from build123d import *

# Parameters (mm, degrees)
F1_DEPTH      = 9
F3_DEPTH      = 25
F4_R          = 4.5
F4_R_2        = 3.5
F5_DEPTH      = 24
F7_DEPTH      = 25
F7_DEPTH_BACK = 25


with BuildPart() as f1:
    # F0 (on Top) → F1 (new body)
    with BuildSketch(Plane.XY):
        Polygon((-3.3, 3.3), (-3.3, 0), (-3.3, -3.3), (0, -3.3), (3.3, -3.3), (3.3, 0), (3.3, 3.3), (0, 3.3), align=None)
        Polygon((6.6, -3.810512), (6.6, 3.810512), (0, 7.621024), (-6.6, 3.810512), (-6.6, -3.810512), (0, -7.621024), align=None)
        Polygon((-3.3, -3.3), (-3.3, 0), (-3.3, 3.3), (0, 3.3), (3.3, 3.3), (3.3, 0), (3.3, -3.3), (0, -3.3), align=None, mode=Mode.SUBTRACT)
    extrude(amount=F1_DEPTH)

    # F2 (on face) → F3 (cut)
    with BuildSketch(Plane(origin=(-6.6, 0, 0), x_dir=(0, -1, 0), z_dir=(-1, 0, 0))):
        with BuildLine():
            ThreePointArc((1.6, -12), (1.131371, -10.868629), (0, -10.4))
            ThreePointArc((0, -10.4), (-1.131371, -13.131371), (1.6, -12))
        make_face()
    extrude(amount=-F3_DEPTH, mode=Mode.SUBTRACT)

    # F4 (on face) → F5 (join)
    with BuildSketch(Plane(origin=(0, 0, 0), x_dir=(1, 0, 0), z_dir=(0, 0, -1))):
        Circle(F4_R)
        Circle(F4_R_2, mode=Mode.SUBTRACT)
    extrude(amount=F5_DEPTH)

    # F6 (on face) → F7 (cut, two sides)
    with BuildSketch(Plane(origin=(0, -3.3, 0), x_dir=(-1, 0, 0), z_dir=(0, 1, 0))) as f7_sk:
        with BuildLine():
            ThreePointArc((0, -16.4), (-1.131371, -19.131371), (1.6, -18))
            ThreePointArc((1.6, -18), (1.131371, -16.868629), (0, -16.4))
        make_face()
    extrude(amount=F7_DEPTH, mode=Mode.SUBTRACT)
    extrude(f7_sk.sketch, amount=-F7_DEPTH_BACK, mode=Mode.SUBTRACT)


solid = f1.part
Model file for the job. Use its own axes, mm. A direction names the side the tool comes from. Coordinates: 2 decimals unless noted, no trailing zeros. Loops run counter-clockwise (first coordinate to the right, second up) from the corner with the lowest first, then second, coordinate; pieces in that order, holes last. Notation, with made-up numbers: (84.25, -17.75) -> (98.25, -17.75) arc R8 cw to (98.25, -12.75) -> close; hole circle Ø11 at (-20.5, 19.25). An arc over 180 degrees is marked (long way). Use one line per item in the form item = value. Start each with the question number.
(1) Cut at C-C on x = -0.5. Give the cut face in (y, z), and give its area (3 significant figures).
(2) Cut at D-D on y = 2.75. Give the cut face in (x, z), and give its area (3 significant figures).
(3) Cut at B-B on z = 4.5. Give the cut face in (x, y).
(4) Flat gauge pins, fed straight in: pin 1 (4 mm diameter, centred on x = 0, y = -2, fed in from -Z); pin 2 (4 mm diameter, centred on x = -3.5, z = -8.5, fed in from -Y); pin 3 (5 mm diameter, centred on x = 0, z = -18, fed in from -Y); pin 4 (8 mm diameter, centred on y = 4, z = -9.5, fed in from +X). Where does each tip first touch, or does it go through?
(5) Tool access for faces 5 (the flat face through (3.3, 0, 4)), 6 (the cylindrical face through (4.292, -1.352, -11.832)), 7 (the flat face through (3.254, -5.742, 4.437)): list every direction of +Z, -Z, +X, -X, +Y, -Y with a clear straight run to the whole face (end or side of a thin tool).
(6) Probe probe 1 along X at (y, z) = (0, -4); probe 2 along X at (y, z) = (1, 3). List the from-to ranges inside material, lowest first. Write a range as from..to.
(7) Cut at A-A on y = 0. Give the cut face in (x, z).
(8) Pull direction X, two halves, no side cores. Call faces 1 (the flat face through (-3.254, 5.742, 4.437)), 2 (the flat face through (3, 3, 0)), 3 (the flat face through (6.6, 0, 4)), 4 (the flat face through (0, 4, -24)): pulls with the +X half, pulls with the -X half, needs draft (parallel to the pull), parting line crosses it, or undercut.
Values:
q1.outline = (-7.33, 0) -> (-4.47, 0) -> (-4.47, -16.48) -> (-3.46, -16.48) -> (-3.46, 0) -> (-3.3, 0) -> (-3.3, 9) -> (-7.33, 9) -> close; (-4.47, -24) -> (-3.46, -24) -> (-3.46, -19.52) -> (-4.47, -19.52) -> close; (3.3, 0) -> (3.46, 0) -> (3.46, -16.48) -> (4.47, -16.48) -> (4.47, 0) -> (7.33, 0) -> (7.33, 9) -> (3.3, 9) -> close; (3.46, -24) -> (4.47, -24) -> (4.47, -19.52) -> (3.46, -19.52) -> close
q1.area = 115 mm2
q2.outline = (-6.6, 0) -> (-3.56, 0) -> (-3.56, -24) -> (-2.17, -24) -> (-2.17, 0) -> (-3.3, 0) -> (-3.3, 9) -> (-6.6, 9) -> close; (2.17, -24) -> (3.56, -24) -> (3.56, 0) -> (6.6, 0) -> (6.6, 9) -> (3.3, 9) -> (3.3, 0) -> (2.17, 0) -> close
q2.area = 126 mm2
q3.outline = (-6.6, -3.81) -> (0, -7.62) -> (6.6, -3.81) -> (6.6, 3.81) -> (0, 7.62) -> (-6.6, 3.81) -> close; hole (-3.3, -3.3) -> (3.3, -3.3) -> (3.3, 3.3) -> (-3.3, 3.3) -> close
q4.pin_1 = -24
q4.pin_2 = -4.24
q4.pin_3 = -4.5
q4.pin_4 = 4.5
q5.face_5 = +Z
q5.face_6 = -Z
q5.face_7 = +Z, -Z, +X, -Y
q6.probe_1 = -4.5..-3.5, 3.5..4.5
q6.probe_2 = -6.6..-3.3, 3.3..6.6
q7.outline = (-6.6, 0) -> (-4.5, 0) -> (-4.5, -24) -> (-3.5, -24) -> (-3.5, 0) -> (-3.3, 0) -> (-3.3, 9) -> (-6.6, 9) -> close; (3.3, 0) -> (3.5, 0) -> (3.5, -24) -> (4.5, -24) -> (4.5, 0) -> (6.6, 0) -> (6.6, 9) -> (3.3, 9) -> close
q8.face_1 = pulls with the -X half
q8.face_2 = undercut
q8.face_3 = pulls with the +X half
q8.face_4 = needs draft
